from build123d import *

# Parameters (mm, degrees)
F0_R     = 1.655877
F0_R_2   = 2.651838
F0_R_3   = 3.310353
F0_R_4   = 2.921
F0_R_5   = 1.545023
F0_R_6   = 1.905
F0_R_7   = 2.289524
F0_R_8   = 2.989225
F0_R_9   = 2.932024
F1_DEPTH = 3.175
F2_W     = 2.54
F2_H     = 2.54
F3_DEPTH = 3.175


with BuildPart() as f1:
    # F0 (on Top) → F1 (new body)
    with BuildSketch(Plane.XY):
        Polygon((32.829497, -3.6195), (24.320502, -0.9525), (19.1135, -3.6195), (15.303499, -2.6035), (7.044703, -6.867298), (2.976148, -13.144501), (2.976148, -16.312003), (0, -13.144501), (0, -17.970501), (1.7145, -23.669264), (8.064501, -31.559501), (4.6355, -31.559501), (11.493499, -36.004499), (14.414499, -34.734499), (21.272501, -36.004499), (27.368499, -33.3375), (27.368499, -37.9095), (29.936647, -35.496499), (36.131501, -30.7975), (36.131501, -28.2575), (38.068253, -25.5905), (38.068253, -22.542501), (39.166847, -23.669264), (40.322501, -22.542501), (42.799, -25.082501), (41.084498, -13.652501), (39.306503, -10.731501), (37.9095, -10.731501), (36.131501, -9.2075), (29.936647, -5.965224), (29.5275, -4.6355), align=None)
        with Locations((12.128499, -29.908501)):
            Circle(F0_R, mode=Mode.SUBTRACT)
        with Locations((17.335502, -31.305499)):
            Circle(F0_R_2, mode=Mode.SUBTRACT)
        with Locations((6.286501, -20.7645)):
            Circle(F0_R_3, mode=Mode.SUBTRACT)
        with BuildLine():
            Line((13.620393, -24.859201), (12.763499, -19.4945))
            Line((12.763499, -19.4945), (14.541501, -21.907501))
            Line((14.541501, -21.907501), (15.829229, -21.3995))
            Line((15.829229, -21.3995), (16.612777, -23.38571))
            Line((16.612777, -23.38571), (18.882671, -22.190495))
            Line((18.882671, -22.190495), (17.496092, -19.557172))
            ThreePointArc((17.496092, -19.557172), (14.764748, -17.393266), (16.065503, -14.160501))
            ThreePointArc((16.065503, -14.160501), (16.325903, -16.779071), (18.732499, -17.8435))
            Line((18.732499, -17.8435), (20.067376, -19.913881))
            Line((20.067376, -19.913881), (23.023179, -17.081501))
            ThreePointArc((23.023179, -17.081501), (25.66988, -16.439906), (27.6225, -14.5415))
            ThreePointArc((27.6225, -14.5415), (26.339514, -19.717253), (21.083658, -20.6175))
            Line((21.083658, -20.6175), (20.067376, -22.190495))
            Line((20.067376, -22.190495), (21.594148, -23.3045))
            Line((21.594148, -23.3045), (22.709592, -22.190495))
            Line((22.709592, -22.190495), (25.418346, -23.809462))
            Line((25.418346, -23.809462), (28.348263, -22.190495))
            Line((28.348263, -22.190495), (25.701909, -26.60206))
            Line((25.701909, -26.60206), (22.7965, -24.859201))
            Line((22.7965, -24.859201), (21.083658, -27.71457))
            Line((21.083658, -27.71457), (18.498735, -24.859201))
            Line((18.498735, -24.859201), (17.318298, -26.60206))
            Line((17.318298, -26.60206), (15.049499, -23.3045))
            Line((15.049499, -23.3045), (13.620393, -24.859201))
        make_face(mode=Mode.SUBTRACT)
        with Locations((30.289499, -28.8925)):
            Circle(F0_R_4, mode=Mode.SUBTRACT)
        with Locations((34.9885, -21.907501)):
            Circle(F0_R_5, mode=Mode.SUBTRACT)
        with Locations((7.048499, -15.0495)):
            Circle(F0_R_6, mode=Mode.SUBTRACT)
        with Locations((13.5255, -7.8105)):
            Circle(F0_R_7, mode=Mode.SUBTRACT)
        with Locations((35.242502, -16.9545)):
            Circle(F0_R_8, mode=Mode.SUBTRACT)
        with Locations((23.558499, -7.4295)):
            Circle(F0_R_9, mode=Mode.SUBTRACT)
    extrude(amount=F1_DEPTH)

    # F2 (on face) → F3 (cut)
    with BuildSketch(Plane.XY.offset(3.175)):
        with Locations((21.902567, -13.187881)):
            Rectangle(F2_W, F2_H)
    extrude(amount=-F3_DEPTH, mode=Mode.SUBTRACT)


solid = f1.part
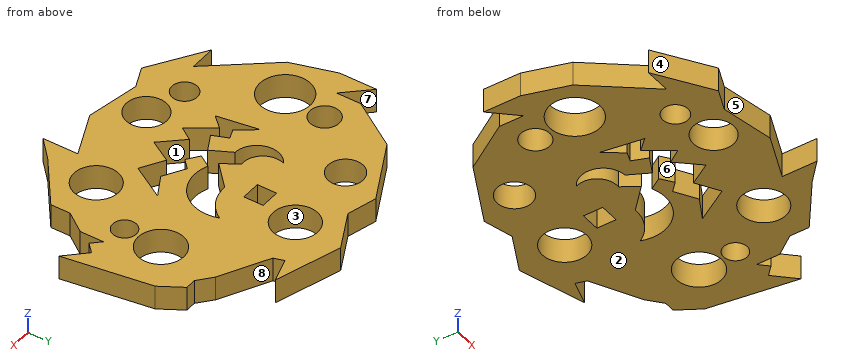
Work out the finished part from the listing and answer in its coordinate system (mm). Face numbers are marked on the shaded views. A direction names the side the tool comes from. Coordinates: 2 decimals unless noted, no trailing zeros. Write each loop counter-clockwise with the first axis right and the second up, starting at its lowest first coordinate (ties: lowest second). Pieces come first, ordered by that corner, then holes.
1. Consider line 1 along Y through (x, z) = (12.5, 1.2); line 2 along X through (y, z) = (-29.5, 0.3); line 3 along Y through (x, z) = (19.5, 0.7). Determine where each line is inside the solid, lowest interval first.
Results list:
line 1: y = -35.57 to -31.52, -28.29 to -9.86, -5.76 to -4.05
line 2: x = 6.41 to 10.52, 13.73 to 15.39, 19.28 to 27.43, 33.15 to 36.13
line 3: y = -35.68 to -32.84, -29.77 to -25.97, -19.03 to -3.42
2. The part is cut by section B-B, the plane x = 7.5. Write down the section's boundary in (y, z) (1 decimal).
Results list:
outline: (-33.4, 0) - (-31.6, 0) - (-31.6, 3.2) - (-33.4, 3.2) - close; (-30.9, 0) - (-23.8, 0) - (-23.8, 3.2) - (-30.9, 3.2) - close; (-17.7, 0) - (-16.9, 0) - (-16.9, 3.2) - (-17.7, 3.2) - close; (-13.2, 0) - (-6.6, 0) - (-6.6, 3.2) - (-13.2, 3.2) - close
3. The part is cut by section C-C, the plane z = 0.9. State how many separate pieces and enclosed holes the cut face has, and give its area (3 significant figures).
Results list:
separate pieces: 1
enclosed holes: 11
area: 792 mm2
4. Flat-ended cylindrical pins translate along their axes: pin 1 (0.8 mm diameter, centred on x = 21.5, z = 2.5, fed in from +Y); pin 2 (5 mm diameter, centred on x = 17.34, y = -31.31, fed in from +Z); pin 3 (1 mm diameter, centred on y = -34.5, z = 1.5, fed in from -X); pin 4 (1.3 mm diameter, centred on x = 22, z = 1, fed in from -Y). Find the tip coordinate at first contact, or state that the pin passes through.
Results list:
pin 1: stops at y = -2.19
pin 2: passes through
pin 3: stops at x = 8.4
pin 4: stops at y = -35.97
5. For a pull along Y with two mould halves and no side action, classify the marked faces 1, 2, 3 and 4 as +Y half, -Y half, draft (parallel to the pull), parting line (faces both ways), or undercut.
Results list:
face 1: undercut
face 2: draft
face 3: undercut
face 4: -Y half
6. The part is cut by section A-A, the plane x = 37. Write down the section's boundary in (y, z) (3 decimals).
Results list:
outline: (-27.062, 0) - (-19.372, 0) - (-19.372, 3.175) - (-27.062, 3.175) - close; (-14.537, 0) - (-9.952, 0) - (-9.952, 3.175) - (-14.537, 3.175) - close
7. For the marked faces 5, 6, 7 and 8, determine the directions among +Z, -Z, +X, -X, +Y, -Y from which every point of the face is accessible in a straight line to the end or side of a thin tool.
Results list:
face 5: +Z, -Z, -Y
face 6: +Z, -Z
face 7: +Z, -Z, +Y
face 8: +Z, -Z, +X
